Build history of the part. All positions in model axes, mm. A direction names the side the tool comes from. Coordinates: 2 decimals unless noted, no trailing zeros. Loops run counter-clockwise (first coordinate to the right, second up) from the corner with the lowest first, then second, coordinate; pieces in that order, holes last. Notation, with made-up numbers: (-12, 59) - (37, 59) arc R35 cw to (37, 97) - close; hole circle Ø7 at (-24.75, -32.75). An arc over 180 degrees is marked (long way). One line per item, written item: value.
```python
from build123d import *

# Parameters (mm, degrees)
SKETCH1_W           = 15
SKETCH1_H           = 13
BOSS_EXTRUDE1_DEPTH = 10.1
SKETCH2_W           = 3.5
SKETCH2_H           = 3
BOSS_EXTRUDE2_DEPTH = 1.3
CUT_EXTRUDE1_REACH  = 21.728
SKETCH4_W           = 6.77
SKETCH4_H           = 5
BOSS_EXTRUDE3_DEPTH = 4.6
SKETCH5_W           = 6.77
SKETCH5_H           = 5
BOSS_EXTRUDE4_DEPTH = 4.6


with BuildPart() as part:
    # Sketch1 → Boss-Extrude1 (new body)
    with BuildSketch(Plane(origin=(0, 0, 0), x_dir=(1, 0, 0), z_dir=(0, 1, 0))):
        with Locations((7.5, 6.5)):
            Rectangle(SKETCH1_W, SKETCH1_H)
    extrude(amount=BOSS_EXTRUDE1_DEPTH)

    # Sketch2 → Boss-Extrude2 (add)
    with BuildSketch(Plane(origin=(0, 10.1, 0), x_dir=(1, 0, 0), z_dir=(0, 1, 0))):
        with Locations((7.75, 1.5)):
            Rectangle(SKETCH2_W, SKETCH2_H)
    extrude(amount=BOSS_EXTRUDE2_DEPTH)

    # Sketch3 → Cut-Extrude1 (cut, up to next)
    with BuildSketch(Plane(origin=(9.5, 0, 0), x_dir=(0, 0, -1), z_dir=(1, 0, 0)), mode=Mode.PRIVATE) as cut_extrude1_sk1:
        Polygon((0, 10.1), (3, 11.4), (0, 11.4), align=None)
    cut_extrude1_tool1 = extrude(cut_extrude1_sk1.sketch, amount=-CUT_EXTRUDE1_REACH, mode=Mode.PRIVATE) & part.part
    add(cut_extrude1_tool1.solids().sort_by_distance((9.5, 10.966667, -1))[0], mode=Mode.SUBTRACT)

    # Sketch4 → Boss-Extrude3 (add)
    with BuildSketch(Plane(origin=(15, 0, 0), x_dir=(0, 0, -1), z_dir=(1, 0, 0))):
        with Locations((9.615, 2.5)):
            Rectangle(SKETCH4_W, SKETCH4_H)
    extrude(amount=BOSS_EXTRUDE3_DEPTH)

    # Sketch5 → Boss-Extrude4 (add)
    with BuildSketch(Plane.ZY):
        with Locations((-9.615, 2.5)):
            Rectangle(SKETCH5_W, SKETCH5_H)
    extrude(amount=BOSS_EXTRUDE4_DEPTH)


solid = part.part
```
Item 1: Drop flat-ended pins along their axis: P1, Ø5, axis at y = 8.5, z = -11.5, coming from the +X side; P2, Ø4, axis at x = 13.5, z = -6.5, coming from the +Y side; P3, Ø2.5, axis at x = 17.5, z = -9.5, coming from the +Y side. Give the stop position or say it passes through.
Check result:
P1: stops at x = 15
P2: stops at y = 10.1
P3: stops at y = 5
Item 2: Cut at C-C, the plane x = 8.75. Write the cut outline in (y, z), then the cut area to 3 significant figures.
Check result:
outline: (0, -13) - (10.1, -13) - (10.1, -3) - (11.4, -3) - (10.1, 0) - (0, 0) - close
area: 133 mm^2
Item 3: Cut at D-D, the plane y = 7.25. Write the cut outline in (x, z), then the cut area to 3 significant figures.
Check result:
outline: (0, -13) - (15, -13) - (15, 0) - (0, 0) - close
area: 195 mm^2
Item 4: Cut at B-B, the plane z = -8.5. Write the cut outline in (x, y), then the cut area to 4 significant figures.
Check result:
outline: (-4.6, 0) - (19.6, 0) - (19.6, 5) - (15, 5) - (15, 10.1) - (0, 10.1) - (0, 5) - (-4.6, 5) - close
area: 197.5 mm^2
Item 5: Tool access for faces 1 (the face through (17, 2, -6.23)), 2 (the face through (17, 5, -10)), 3 (the face through (6, 10.5, -2.1)), 4 (the face through (8, 11, -3)): list every direction of +Z, -Z, +X, -X, +Y, -Y with a clear straight run to the whole face (end or side of a thin tool).
Check result:
face 1: +Z, +X, +Y, -Y
face 2: +Z, -Z, +X, +Y
face 3: +Z, -Z, -X, +Y
face 4: -Z, +X, -X, +Y
Item 6: Probe probe 1 along X at (y, z) = (9.25, -5); probe 2 along Z at (x, y) = (16.5, 2.75); probe 3 along Y at (x, z) = (1, -10.25). List the from-to ranges inside material, lowest first. Write a range as from..to.
Check result:
probe 1: x = 0..15
probe 2: z = -13..-6.23
probe 3: y = 0..10.1
Item 7: Cut at A-A, the plane y = 3.25. Write the cut outline in (x, z), then the cut area to 3 significant figures.
Check result:
outline: (-4.6, -13) - (19.6, -13) - (19.6, -6.23) - (15, -6.23) - (15, 0) - (0, 0) - (0, -6.23) - (-4.6, -6.23) - close
area: 257 mm^2
